from build123d import *

# Parameters (mm, degrees)
BOSS_EXTRUDE1_DEPTH = 3.175
SKETCH4_W           = 3.175
SKETCH4_H           = 4
CUT_EXTRUDE1_DEPTH  = 10
BOSS_EXTRUDE2_DEPTH = 3.175


with BuildPart() as part:
    # Sketch2 → Boss-Extrude1 (new body)
    with BuildSketch(Plane.XY):
        Polygon((-2, 17.975), (-2, 21.15), (-9.5, 21.15), (-9.5, 17.975), (-13.5, 17.975), (-13.5, 21.15), (-21.15, 21.15), (-21.15, 13.5), (-17.975, 13.5), (-17.975, 9.5), (-21.15, 9.5), (-21.15, 2), (-17.975, 2), (-17.975, -2), (-21.15, -2), (-21.15, -9.5), (-17.975, -9.5), (-17.975, -13.5), (-21.15, -13.5), (-21.15, -21.15), (-13.5, -21.15), (-13.5, -17.975), (-9.5, -17.975), (-9.5, -21.15), (-2, -21.15), (-2, -17.975), (2, -17.975), (2, -21.15), (9.5, -21.15), (9.5, -17.975), (13.5, -17.975), (13.5, -21.15), (17.975, -21.15), (17.975, -13.5), (21.15, -13.5), (21.15, -9.5), (17.975, -9.5), (17.975, -2), (21.15, -2), (21.15, 2), (17.975, 2), (17.975, 9.5), (21.15, 9.5), (21.15, 13.5), (17.975, 13.5), (17.975, 21.15), (13.5, 21.15), (13.5, 17.975), (9.5, 17.975), (9.5, 21.15), (2, 21.15), (2, 17.975), align=None)
    extrude(amount=BOSS_EXTRUDE1_DEPTH)

    # Sketch4 → Cut-Extrude1 (cut)
    with BuildSketch(Plane.XY.offset(3.175)):
        Polygon((-13.5, 13.5), (-13.5, 17.975), (-13.5, 21.15), (-21.15, 21.15), (-21.15, -21.15), (-13.5, -21.15), (-13.5, -17.975), (-13.5, -13.5), (-13.5, -9.5), (-13.5, -2), (-13.5, 2), (-13.5, 9.5), align=None)
        with Locations((-11.9125, 11.5)):
            Rectangle(SKETCH4_W, SKETCH4_H)
        with Locations((-11.9125, 0)):
            Rectangle(SKETCH4_W, SKETCH4_H)
        with Locations((-11.9125, -11.5)):
            Rectangle(SKETCH4_W, SKETCH4_H)
    extrude(amount=-CUT_EXTRUDE1_DEPTH, mode=Mode.SUBTRACT)

    # Sketch3 → Boss-Extrude2 (add)
    with BuildSketch(Plane.XY.offset(3.175)):
        Polygon((-13.54064, 18.01564), (-13.54064, 13.45936), (-10.36564, 13.45936), (-10.36564, 9.54064), (-13.54064, 9.54064), (-13.54064, 1.95936), (-10.36564, 1.95936), (-10.36564, -1.95936), (-13.54064, -1.95936), (-13.54064, -9.54064), (-10.36564, -9.54064), (-10.36564, -13.45936), (-13.54064, -13.45936), (-13.54064, -18.01564), (-9.54064, -18.01564), (-9.54064, -21.19064), (-1.95936, -21.19064), (-1.95936, -18.01564), (1.95936, -18.01564), (1.95936, -21.19064), (9.54064, -21.19064), (9.54064, -18.01564), (13.45936, -18.01564), (13.45936, -21.19064), (18.01564, -21.19064), (18.01564, -13.54064), (21.19064, -13.54064), (21.19064, -9.45936), (18.01564, -9.45936), (18.01564, -2.04064), (21.19064, -2.04064), (21.19064, 2.04064), (18.01564, 2.04064), (18.01564, 9.45936), (21.19064, 9.45936), (21.19064, 13.54064), (18.01564, 13.54064), (18.01564, 21.19064), (13.45936, 21.19064), (13.45936, 18.01564), (9.54064, 18.01564), (9.54064, 21.19064), (1.95936, 21.19064), (1.95936, 18.01564), (-1.95936, 18.01564), (-1.95936, 21.19064), (-9.54064, 21.19064), (-9.54064, 18.01564), align=None)
    extrude(amount=-BOSS_EXTRUDE2_DEPTH)


solid = part.part
Design review of the part built by this model. Coordinates are the model's own, in mm. A direction names the side the tool comes from. Coordinates: 2 decimals unless noted, no trailing zeros. Order: outer loops, then holes, each group sorted by start corner. A loop starts at its lowest first (then second) coordinate and runs counter-clockwise, first axis right, second up. Notation, with made-up numbers: M 59,26 L 82,26 A28 ccw 82,59 Z; hole C -6,47 d6. An arc over 180 degrees is marked long. Use a Markdown table: item, result.
(1) For P1, Ø1.6, axis at x = 20, z = 1, coming from the -Y side; P2, Ø1, axis at x = 10.5, z = 2, coming from the -Y side; P3, Ø1, axis at x = 19.5, z = 1.5, coming from the +Y side, all flat-tipped, find the tip position at first contact; note any pin that passes through.
Worked answers:
| item | result |
|---|---|
| P1 | stops at y = -13.54 |
| P2 | stops at y = -18.02 |
| P3 | stops at y = 13.54 |
(2) Add section B-B (y = -5). Give the boundary of the cut face in (x, z) (3 decimals).
Worked answers:
| item | result |
|---|---|
| outline | M -13.541,0 L 18.016,0 L 18.016,3.175 L -13.541,3.175 Z |
(3) Wall thickness on probe 1 along X at (y, z) = (19.5, 0.55); probe 2 along X at (y, z) = (-6, 0.3); probe 3 along Y at (x, z) = (1.5, 2.5): over which ranges is each line inside the solid? List them lowest first.
Worked answers:
| item | result |
|---|---|
| probe 1 | x = -9.54 to -1.96, 1.96 to 9.54, 13.46 to 18.02 |
| probe 2 | x = -13.54 to 18.02 |
| probe 3 | y = -18.02 to 18.02 |
(4) Add section C-C (x = 11). Give the boundary of the cut face in (y, z) (3 decimals).
Worked answers:
| item | result |
|---|---|
| outline | M -18.016,0 L 18.016,0 L 18.016,3.175 L -18.016,3.175 Z |
(5) Draft analysis for pull direction Y (two halves, no side actions). For faces 4 (the flat face through (6, -21.191, 2)), 5 (the flat face through (-12, -13.459, 2)), 6 (the flat face through (18.016, 17, 2)), state which applies: released by +Y, released by -Y, zero draft, split by the parting line, or undercut.
Worked answers:
| item | result |
|---|---|
| face 4 | released by -Y |
| face 5 | undercut |
| face 6 | zero draft |
(6) For faces 1 (the flat face through (20, 13.541, 2)), 2 (the flat face through (-1.959, -20, 2)), 3 (the flat face through (0, 18.016, 2)), list the 3-axis set-ups (+Z, -Z, +X, -X, +Y, -Y) from which the entire face can be reached by the end or side of a thin tool; tool diameter is ignored.
Worked answers:
| item | result |
|---|---|
| face 1 | +Z, -Z, +X, +Y |
| face 2 | +Z, -Z, -Y |
| face 3 | +Z, -Z, +Y |
(7) Add section A-A (x = 19). Give the boundary of the cut face in (y, z) (3 decimals), then the cut area to 3 significant figures.
Worked answers:
| item | result |
|---|---|
| outline | M -13.541,0 L -9.459,0 L -9.459,3.175 L -13.541,3.175 Z; M -2.041,0 L 2.041,0 L 2.041,3.175 L -2.041,3.175 Z; M 9.459,0 L 13.541,0 L 13.541,3.175 L 9.459,3.175 Z |
| area | 38.9 mm2 |
